Geometry check sheet. Reference: drawing and pictorial views, mm from the part's lowest x, y, z. A direction names the side the tool comes from. Round coordinates to 2 decimals unless told otherwise and drop trailing zeros. Write each loop counter-clockwise with the first axis right and the second up, starting at its lowest first coordinate (ties: lowest second). Pieces come first, ordered by that corner, then holes. Notation, with made-up numbers: (-24, -24.75) -> (1, -24.75) arc R16 cw to (1, -13.75) -> close; hole circle Ø9 at (1, 21). An arc over 180 degrees is marked (long way). Write item = value, one per line.
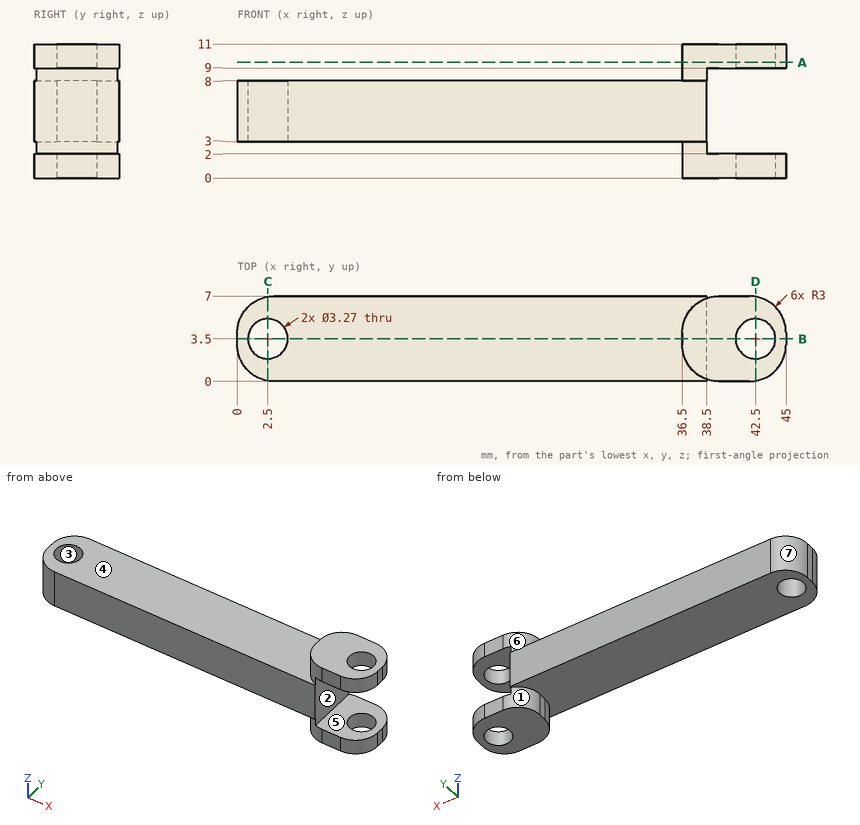
(1) Sectioned sample at D-D on x = 42.5. Enter the section's corners in (y, z) (3 decimals).
Worked answers:
outline = (0.042, 0) -> (1.865, 0) -> (1.865, 2) -> (0.042, 2) -> close; (0.042, 9) -> (1.865, 9) -> (1.865, 11) -> (0.042, 11) -> close; (5.135, 0) -> (6.958, 0) -> (6.958, 2) -> (5.135, 2) -> close; (5.135, 9) -> (6.958, 9) -> (6.958, 11) -> (5.135, 11) -> close
(2) Sectioned sample at B-B on y = 3.5. Enter the section's corners in (x, z) (3 decimals), then the cut area to 3 significant figures.
Worked answers:
outline = (0, 3) -> (0.865, 3) -> (0.865, 8) -> (0, 8) -> close; (4.135, 3) -> (36.5, 3) -> (36.5, 0) -> (40.865, 0) -> (40.865, 2) -> (38.5, 2) -> (38.5, 9) -> (40.865, 9) -> (40.865, 11) -> (36.5, 11) -> (36.5, 8) -> (4.135, 8) -> close; (44.135, 0) -> (45, 0) -> (45, 2) -> (44.135, 2) -> close; (44.135, 9) -> (45, 9) -> (45, 11) -> (44.135, 11) -> close
area = 201 mm²
(3) Access from +Z, -Z, +X, -X, +Y, -Y to the whole of each face (thin tool, end or side, straight path). Record for the marked faces 5, 6 and 7.
Worked answers:
face_5 = +X, +Y, -Y
face_6 = +Z, -X, +Y
face_7 = +Z, -Z, -X, +Y
(4) Go/stop test with flat-tipped pins: P1, Ø1.5, axis at y = 2, z = 6.5, coming from the +X side; P2, Ø1.1, axis at y = 3.5, z = 1.5, coming from the -X side; P3, Ø3.5, axis at x = 16.5, y = 3.5, coming from the -Z side. Record where each tip stops, or that it passes through.
Worked answers:
P1 = 38.5
P2 = 36.5
P3 = 3
(5) Sectioned sample at A-A on z = 9.5. Enter the section's corners in (x, y) (3 decimals), then the cut area to 3 significant figures.
Worked answers:
outline = (36.5, 3) arc R3 ccw to (39.5, 0) -> (42, 0) arc R3 ccw to (45, 3) -> (45, 4) arc R3 ccw to (42, 7) -> (39.5, 7) arc R3 ccw to (36.5, 4) -> close; hole circle Ø3.27 at (42.5, 3.5)
area = 43.4 mm²
(6) Sectioned sample at C-C on x = 2.5. Enter the section's corners in (y, z) (3 decimals), then the cut area to 3 significant figures.
Worked answers:
outline = (0.042, 3) -> (1.865, 3) -> (1.865, 8) -> (0.042, 8) -> close; (5.135, 3) -> (6.958, 3) -> (6.958, 8) -> (5.135, 8) -> close
area = 18.2 mm²
(7) Material ranges on L1, parallel to Z at x = 28, y = 5; L2, parallel to Z at x = 41.5, y = 1.5; L3, parallel to Y at x = 2.5, z = 5.6 (3 decimals), recorded low to high. Write a range as [from, to].
Worked answers:
L1 = [3, 8]
L2 = [0, 2], [9, 11]
L3 = [0.042, 1.865], [5.135, 6.958]
(8) Release check for a two-part mould opening along X. For the marked faces 1, 2, 3 and 4 record: pulls with the +X half, pulls with the -X half, needs draft (parallel to the pull), parting line crosses it, or undercut.
Worked answers:
face_1 = pulls with the -X half
face_2 = pulls with the +X half
face_3 = undercut
face_4 = needs draft
